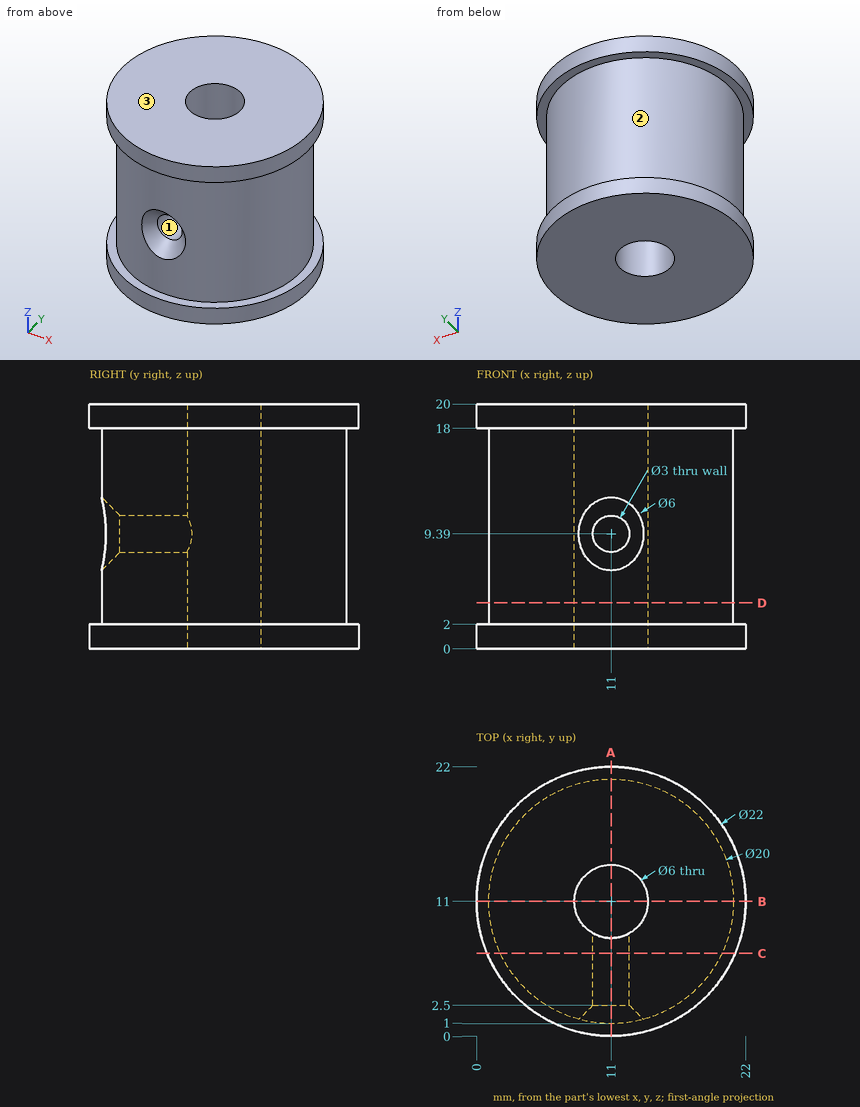
Here's the drawing with two shaded views (mm, measured from the low corner). I have some questions. Coordinates: 2 decimals unless noted, no trailing zeros. Order: outer loops, then holes, each group sorted by start corner. A loop starts at its lowest first (then second) coordinate and runs counter-clockwise, first axis right, second up.
Q1. Please list where these lines run through material, in increasing order: L1, parallel to Z at x = 11, y = 6.3; L2, parallel to Y at x = 11, z = 4.75; L3, parallel to Y at x = 13.25, z = 5 (1 decimal).
Q2. Will these pins go through, and if not, where does the flat tip stop? pin 1 (1.5 mm diameter, centred on x = 15.5, z = 13, fed in from -Y); pin 2 (1 mm diameter, centred on y = 18.5, z = 15.5, fed in from +X); pin 3 (1 mm diameter, centred on y = 13, z = 17, fed in from +X); pin 4 (3.5 mm diameter, centred on x = 11, y = 11, fed in from -Z).
Q3. Suppose I cut it at D-D on z = 3.75. Please give me the cut outline in (x, y), and give its area (3 significant figures).
Q4. Suppose I cut it at B-B on y = 11. Please give me the cut outline in (x, z), and give its area (3 significant figures).
Q5. Suppose I cut it at C-C on y = 6.75. Please give me the cut outline in (x, z).
Q6. Thinking about a two-plate mould opening in X: for the marked faces 1, 2 and 3, which applies, released by +X, released by -X, zero draft, split by the parting line, or undercut?
Q7. Suppose I cut it at A-A on x = 11. Please give me the cut outline in (y, z), and give its area (3 significant figures).
Answer:
1. L1: z = 0 to 7.89, 10.89 to 20
1. L2: y = 1 to 8, 14 to 21
1. L3: y = 1.3 to 9, 13 to 20.7
2. pin 1: stops at y = 1.73
2. pin 2: stops at x = 18.14
2. pin 3: stops at x = 20.89
2. pin 4: passes through
3. outline: circle Ø20 at (11, 11); hole circle Ø6 at (11, 11)
3. area: 286 mm2
4. outline: (0, 0) - (8, 0) - (8, 20) - (0, 20) - (0, 18) - (1, 18) - (1, 2) - (0, 2) - close; (14, 0) - (22, 0) - (22, 2) - (21, 2) - (21, 18) - (22, 18) - (22, 20) - (14, 20) - close
4. area: 288 mm2
5. outline: (0.85, 0) - (21.15, 0) - (21.15, 2) - (20.05, 2) - (20.05, 18) - (21.15, 18) - (21.15, 20) - (0.85, 20) - (0.85, 18) - (1.95, 18) - (1.95, 2) - (0.85, 2) - close; hole circle Ø3 at (11, 9.39)
6. face 1: undercut
6. face 2: split by the parting line
6. face 3: zero draft
7. outline: (0, 0) - (8, 0) - (8, 7.89) - (2.5, 7.89) - (1, 6.39) - (1, 2) - (0, 2) - close; (0, 18) - (1, 18) - (1, 12.39) - (2.5, 10.89) - (8, 10.89) - (8, 20) - (0, 20) - close; (14, 0) - (22, 0) - (22, 2) - (21, 2) - (21, 18) - (22, 18) - (22, 20) - (14, 20) - close
7. area: 265 mm2
